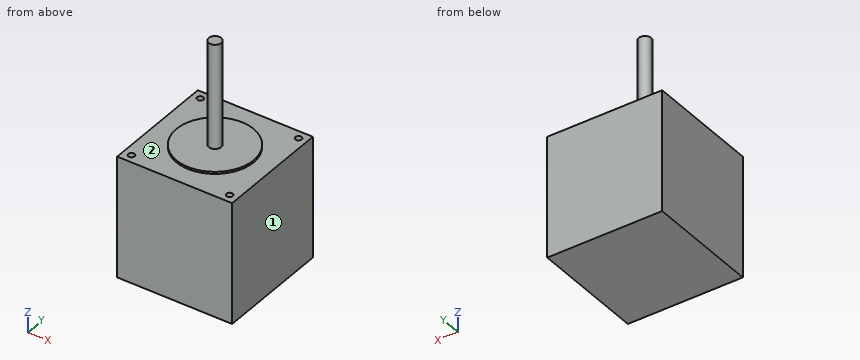
```python
from build123d import *

# Parameters (mm, degrees)
F0_W     = 55
F0_H     = 55
F1_DEPTH = 58
F2_R     = 18.5
F3_DEPTH = 1
F4_R     = 3
F5_DEPTH = 50
F6_R     = 1.5
F7_DEPTH = 25


with BuildPart() as f1:
    # F0 (on Top) → F1 (new body)
    with BuildSketch(Plane.XY):
        with Locations((27.5, 27.5)):
            Rectangle(F0_W, F0_H)
    extrude(amount=F1_DEPTH)

    # F2 (on face) → F3 (join)
    with BuildSketch(Plane.XY.offset(58)):
        with Locations((27.5, 27.5)):
            Circle(F2_R)
    extrude(amount=F3_DEPTH)

    # F4 (on face) → F5 (join)
    with BuildSketch(Plane.XY.offset(59)):
        with Locations((27.5, 27.5)):
            Circle(F4_R)
    extrude(amount=F5_DEPTH)

    # F6 (on face) → F7 (cut)
    with BuildSketch(Plane.XY.offset(58)):
        with Locations((4, 51)):
            Circle(F6_R)
        with Locations((4, 4)):
            Circle(F6_R)
        with Locations((51, 4)):
            Circle(F6_R)
        with Locations((51, 51)):
            Circle(F6_R)
    extrude(amount=-F7_DEPTH, mode=Mode.SUBTRACT)


solid = f1.part
```
Here's how the part is built. I have some questions about the finished solid (model axes, mm). Face numbers are marked on the shaded views. A direction names the side the tool comes from. Give positions to 0.01 mm unless a question says otherwise; leave off trailing zeros. Write each loop counter-clockwise with the first axis right and the second up, starting at its lowest first coordinate (ties: lowest second). Pieces come first, ordered by that corner, then holes. Notation, with made-up numbers: (29.25, 5) -> (68.25, 5) arc R17 ccw to (68.25, 11) -> close; hole circle Ø9 at (-25.5, 69.25). An arc over 180 degrees is marked (long way). Use one line per item in the form item = value.
1) If I drill on L1, parallel to Y at x = 51, z = 46; L2, parallel to Z at x = 52.5, y = 44; L3, parallel to Z at x = 42, y = 18.5, over which ranges is the centre line in solid material (lowest first)? Write a range as [from, to].
Verdict:
L1 = [0, 2.5], [5.5, 49.5], [52.5, 55]
L2 = [0, 58]
L3 = [0, 59]
2) Suppose I cut it at A-A (y = 21.5). Please give me the cut outline in (x, z), and give its area (4 significant figures).
Verdict:
outline = (0, 0) -> (55, 0) -> (55, 58) -> (45, 58) -> (45, 59) -> (10, 59) -> (10, 58) -> (0, 58) -> close
area = 3,225 mm2
3) I'm going to push flat-ended pins straight in: pin 1 (3.5 mm diameter, centred on x = 4, y = 51, fed in from +Z); pin 2 (2.5 mm diameter, centred on x = 51, y = 51, fed in from +Z); pin 3 (6 mm diameter, centred on y = 26, z = 92.5, fed in from -X). Where does each tip first touch, or does it pass through?
Verdict:
pin_1 = 58
pin_2 = 33
pin_3 = 24.5
4) Suppose I cut it at D-D (z = 83). Please give me the cut outline in (x, y), and give its area (3 significant figures).
Verdict:
outline = circle Ø6 at (27.5, 27.5)
area = 28.3 mm2
5) Suppose I cut it at B-B (x = 51). Please give me the cut outline in (y, z).
Verdict:
outline = (0, 0) -> (55, 0) -> (55, 58) -> (52.5, 58) -> (52.5, 33) -> (49.5, 33) -> (49.5, 58) -> (5.5, 58) -> (5.5, 33) -> (2.5, 33) -> (2.5, 58) -> (0, 58) -> close
6) On a 3-axis mill with a long thin cutter (end or side, diameter ignored), from which of +Z, -Z, +X, -X, +Y, -Y can I reach the whole of each face in a straight line? I mean the marked faces 1 and 2. Say none if no direction works.
Verdict:
face_1 = +Z, -Z, +X, +Y, -Y
face_2 = +Z
